from build123d import *

# Parameters (mm, degrees)
SKETCH_1_W          = 10
SKETCH_1_H          = 12
EXTRUDE_1_DEPTH     = 6
SKETCH_2_R          = 1
CUT_EXTRUDE_1_DEPTH = 17.733200531
SKETCH_2_3_R        = 2
CUT_EXTRUDE_2_DEPTH = 4
SKETCH_3_R          = 2
CUT_EXTRUDE_3_DEPTH = 17.733200531
SKETCH_4_W          = 5.2
SKETCH_4_H          = 3.5
CUT_EXTRUDE_4_DEPTH = 4
SKETCH_6_R          = 0.7
CUT_EXTRUDE_5_DEPTH = 17.733200531
SKETCH_6_3_R        = 1
CUT_EXTRUDE_6_DEPTH = 0.9
CUT_EXTRUDE_START   = -9.1
SKETCH_6_4_R        = 1
CUT_EXTRUDE_7_DEPTH = 0.9
SKETCH_7_W          = 10
SKETCH_7_H          = 6
EXTRUDE_3_DEPTH     = 3
SKETCH_8_R          = 0.6
CUT_EXTRUDE_8_DEPTH = 20


with BuildPart() as part:
    # 草图1 → 凸台-拉伸1 (new body)
    with BuildSketch(Plane(origin=(0, 0, 0), x_dir=(1, 0, 0), z_dir=(0, 1, 0))):
        with Locations((5, -6)):
            Rectangle(SKETCH_1_W, SKETCH_1_H)
    extrude(amount=EXTRUDE_1_DEPTH)

    # 草图2 → 切除-拉伸1 (cut, through all)
    with BuildSketch(Plane(origin=(0, 6, 0), x_dir=(1, 0, 0), z_dir=(0, 1, 0))):
        with Locations(Location((5, -1.5, 0), (0, 0, 270))):
            Circle(SKETCH_2_R)
        with Locations(Location((5, -10.5, 0), (0, 0, 270))):
            Circle(SKETCH_2_R)
    extrude(amount=-CUT_EXTRUDE_1_DEPTH, mode=Mode.SUBTRACT)

    # 草图2<3> → 切除-拉伸2 (cut)
    with BuildSketch(Plane(origin=(0, 6, 0), x_dir=(1, 0, 0), z_dir=(0, 1, 0))):
        with Locations((5, -1.5)):
            Circle(SKETCH_2_3_R)
        with Locations((5, -10.5)):
            Circle(SKETCH_2_3_R)
    extrude(amount=-CUT_EXTRUDE_2_DEPTH, mode=Mode.SUBTRACT)

    # 草图3 → 切除-拉伸3 (cut, through all)
    with BuildSketch(Plane(origin=(0, 6, 0), x_dir=(1, 0, 0), z_dir=(0, 1, 0))):
        with Locations(Location((5, -6, 0), (0, 0, 270))):
            Circle(SKETCH_3_R)
    extrude(amount=-CUT_EXTRUDE_3_DEPTH, mode=Mode.SUBTRACT)

    # 草图4 → 切除-拉伸4 (cut)
    with BuildSketch(Plane(origin=(0, 6, 0), x_dir=(1, 0, 0), z_dir=(0, 1, 0))):
        with Locations((5, -1.75)):
            Rectangle(SKETCH_4_W, SKETCH_4_H)
        with Locations((5, -10.25)):
            Rectangle(SKETCH_4_W, SKETCH_4_H)
    extrude(amount=-CUT_EXTRUDE_4_DEPTH, mode=Mode.SUBTRACT)

    # 草图6 → 切除-拉伸5 (cut, through all)
    with BuildSketch(Plane.ZY):
        with Locations((1.7, 4.05)):
            Circle(SKETCH_6_R)
        with Locations((10.3, 4.05)):
            Circle(SKETCH_6_R)
    extrude(amount=-CUT_EXTRUDE_5_DEPTH, mode=Mode.SUBTRACT)

    # 草图6<3> → 切除-拉伸6 (cut)
    with BuildSketch(Plane.ZY):
        with Locations((1.7, 4.05)):
            Circle(SKETCH_6_3_R)
        with Locations((10.3, 4.05)):
            Circle(SKETCH_6_3_R)
    extrude(amount=-CUT_EXTRUDE_6_DEPTH, mode=Mode.SUBTRACT)

    # 草图6<4> → 切除-拉伸7 (cut)
    with BuildSketch(Plane.ZY.offset(CUT_EXTRUDE_START)):
        with Locations((1.7, 4.05)):
            Circle(SKETCH_6_4_R)
        with Locations((10.3, 4.05)):
            Circle(SKETCH_6_4_R)
    extrude(amount=-CUT_EXTRUDE_7_DEPTH, mode=Mode.SUBTRACT)

    # 草图7 → 凸台-拉伸3 (add)
    with BuildSketch(Plane.XY.offset(12)):
        with Locations((5, 3)):
            Rectangle(SKETCH_7_W, SKETCH_7_H)
    extrude(amount=EXTRUDE_3_DEPTH)

    # 草图8 → 切除-拉伸8 (cut, through all)
    with BuildSketch(Plane(origin=(10, 0, 0), x_dir=(0, 0, -1), z_dir=(1, 0, 0))):
        with Locations((-13.5, 2.951438323)):
            Circle(SKETCH_8_R)
    extrude(amount=-CUT_EXTRUDE_8_DEPTH, mode=Mode.SUBTRACT)


solid = part.part
CAD build for the part. Positions are in the model's coordinates, mm. A direction names the side the tool comes from. Round coordinates to 2 decimals unless told otherwise and drop trailing zeros. Loops run counter-clockwise (first coordinate to the right, second up) from the corner with the lowest first, then second, coordinate; pieces in that order, holes last. Notation, with made-up numbers: M 48,40.5 L 81,40.5 A15 cw 81,67.5 Z; hole C 7.25,52 d8. An arc over 180 degrees is marked long. One line per question, with ' | ' between items. Start each with the question number.
Item 1: Cut at D-D, the plane x = 4.25. Write the cut outline in (y, z).
Item 2: Cut at B-B, the plane x = 3.25. Write the cut outline in (y, z), plus the area to 4 significant figures.
Item 3: Pin check, flat tips, straight feed: pin 1 Ø1.8 at (y, z) = (4.05, 10.3) entering from +X; pin 2 Ø3 at (x, y) = (5, 4) entering from -Z; pin 3 Ø1 at (y, z) = (4, 2) entering from -X. Stop position of each tip, or through.
Item 4: Two-plate mould, pull along Y, no slides. Class faces 1 (the cylindrical face through (8.34, 4.52, 9.78)), 2 (the flat face through (3, 6, 7)), 3 (the flat face through (5, 3, 15)): pulls with the +Y half, pulls with the -Y half, needs draft (parallel to the pull), parting line crosses it, or undercut.
Item 5: Which spindle directions (+Z, -Z, +X, -X, +Y, -Y) get a long thin tool onto all of the face, cutting with end or side? Do faces 4 (the cylindrical face through (9.544, 3.667, 2.624)), 5 (the flat face through (5, 4, 3.5)), 6 (the flat face through (5, 4, 12)). Say none if no direction does.
Item 6: Cut at A-A, the plane z = 13.5. Write the cut outline in (x, y).
Item 7: Wall check: line 1 (X direction, y = 5.2, z = 1.5); line 2 (X direction, y = 1.1, z = 1.5); line 3 (Y direction, x = 8.1, z = 10.3). Give the ranges that are in metal, low to high.
Item 8: Cut at C-C, the plane y = 1.3. Write the cut outline in (x, z).
Responses:
1) outline: M 0,0 L 2,0 L 2,0.84 L 0,0.84 Z; M 0,2.16 L 2,2.16 L 2,3.5 L 6,3.5 L 6,4.15 L 0,4.15 Z; M 0,7.85 L 6,7.85 L 6,8.5 L 2,8.5 L 2,9.84 L 0,9.84 Z; M 0,11.16 L 2,11.16 L 2,12 L 6,12 L 6,15 L 0,15 Z; hole C 2.95,13.5 d1.2
2) outline: M 0,0 L 2,0 L 2,3.5 L 6,3.5 L 6,5.03 L 0,5.03 Z; M 0,6.97 L 6,6.97 L 6,8.5 L 2,8.5 L 2,12 L 6,12 L 6,15 L 0,15 Z; hole C 2.95,13.5 d1.2 | area: 49.25 mm²
3) pin 1: stops at x = 9.1 | pin 2: stops at z = 3.5 | pin 3: stops at x = 0.9
4) face 1: undercut | face 2: pulls with the +Y half | face 3: needs draft
5) face 4: +X | face 5: -Z, +Y | face 6: +Y
6) outline: M 0,0 L 10,0 L 10,2.35 L 0,2.35 Z; M 0,3.55 L 10,3.55 L 10,6 L 0,6 Z
7) line 1: x = 0 to 2.4, 7.6 to 10 | line 2: x = 0 to 4, 6 to 10 | line 3: y = 0 to 3.35, 4.75 to 6
8) outline: M 0,0 L 10,0 L 10,15 L 0,15 Z; hole C 5,6 d4; hole C 5,1.5 d2; hole C 5,10.5 d2
